For this review, use the dimensioned drawing (mm, ordinates from the lowest corner) and the shaded views. A direction names the side the tool comes from. Round coordinates to 2 decimals unless told otherwise and drop trailing zeros. Write each question's results on one line, items separated by ' | '. Start each with the question number.
Item 1: Add section A-A (z = 12.7). Count the separate pieces of the cut face and the enclosed holes in it.
Item 2: Clearance check with flat-ended pins moving along their axes: pin 1 (4 mm diameter, centred on y = 6.35, z = 33.02, fed in from +X); pin 2 (8 mm diameter, centred on y = 10.5, z = 10.5, fed in from +X); pin 3 (0.7 mm diameter, centred on x = 5.5, y = 5.5, fed in from -Z); pin 4 (5 mm diameter, centred on y = 5.08, z = 12.7, fed in from -X) (1 decimal). State where each tip first meets the part, or that it passes through.
Item 3: The part is to be moulded in two halves that separate along Z. For the marked faces 1, 2 and 3, say which applies: +Z half, -Z half, draft (parallel to the pull), parting line (faces both ways), or undercut.
Item 4: Tool access review of the marked faces 4 and 5: name each direction out of +Z, -Z, +X, -X, +Y, -Y from which nothing blocks a thin tool from reaching the whole face with its end or side.
Item 5: To check wall thickness, follow line 1 along Y through (x, z) = (3.9, 12.7); line 2 along Y through (x, z) = (4.1, 45.72); line 3 along Z through (x, y) = (0.6, 14.5) (1 decimal). State the ranges of each line that lie inside material, in increasing order.
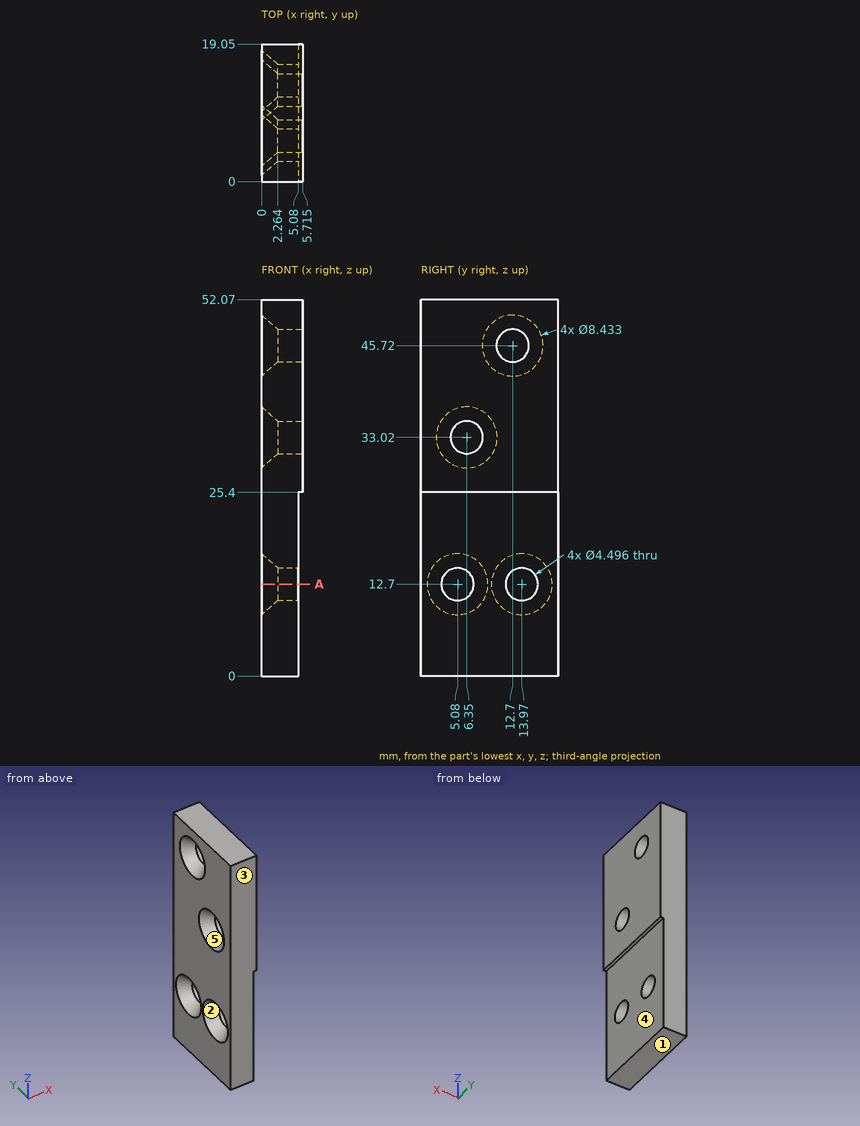
Responses:
1) separate pieces: 3 | enclosed holes: 0
2) pin 1: passes through | pin 2: stops at x = 5.08 | pin 3: stops at z = 25.4 | pin 4: stops at x = 2
3) face 1: -Z half | face 2: undercut | face 3: draft
4) face 4: -Z, +X, +Y, -Y | face 5: -X
5) line 1: y = 0 to 2.83, 7.33 to 11.72, 16.22 to 19.05 | line 2: y = 0 to 10.45, 14.95 to 19.05 | line 3: z = 0 to 9, 16.4 to 42.5, 48.9 to 52.1
